Geometry: final body of the model. Coordinates: model frame, mm. A direction names the side the tool comes from. Give positions to 0.01 mm unless a question says otherwise; leave off trailing zeros. Write each loop counter-clockwise with the first axis right and the second up, starting at its lowest first coordinate (ties: lowest second). Pieces come first, ordered by that corner, then holes. Notation, with made-up numbers: M 7.5,-24 L 14.5,-24 A16 cw 14.5,0 Z; hole C -37,59.25 d3. An arc over 180 degrees is marked long. Answer as a JSON object with one key per item and string values.
from build123d import *

# Parameters (mm, degrees)
F0_R      = 14
F1_DEPTH  = 27.75
F5_R      = 4.45
F6_DEPTH  = 2
F7_R      = 1.55
F8_DEPTH  = 5.6
F9_R      = 4.5
F12_DEPTH = 4.7
F13_R     = 1.5
F14_DEPTH = 4.2
F15_R     = 1
F16_DEPTH = 5.5


with BuildPart() as f1:
    # F0 (on Top) → F1 (new body)
    with BuildSketch(Plane.XY):
        Circle(F0_R)
    extrude(amount=F1_DEPTH)

    # F3 (on Front) → F4 (revolve, cut)
    with BuildSketch(Plane.XZ):
        Polygon((14, 27.75), (9.375, 27.75), (14, 22), align=None)
    revolve(axis=Axis((0, 0, 13.875), (0, 0, -1)), mode=Mode.SUBTRACT)

    # F5 (on face) → F6 (join)
    with BuildSketch(Plane.XY.offset(27.75)):
        Circle(F5_R)
    extrude(amount=F6_DEPTH)

    # F7 (on face) → F8 (join)
    with BuildSketch(Plane.XY.offset(29.75)):
        Circle(F7_R)
    extrude(amount=F8_DEPTH)

    # F10 (on Front) → F11 (revolve, cut)
    with BuildSketch(Plane.XZ):
        Polygon((14, 0), (14, 4.1), (12.375, 0), align=None)
    revolve(axis=Axis((0, 0, 13.875), (0, 0, -1)), mode=Mode.SUBTRACT)

    # F9 (on face) → F12 (cut)
    with BuildSketch(Plane(origin=(0, 0, 0), x_dir=(1, 0, 0), z_dir=(0, 0, -1))):
        Circle(F9_R)
    extrude(amount=-F12_DEPTH, mode=Mode.SUBTRACT)

    # F13 (on face) → F14 (cut)
    with BuildSketch(Plane(origin=(0, 0, 0), x_dir=(1, 0, 0), z_dir=(0, 0, -1))):
        with Locations((-5.656854, 5.656854)):
            Circle(F13_R)
        with Locations((6.717514, 6.717514)):
            Circle(F13_R)
        with Locations((5.656854, -5.656854)):
            Circle(F13_R)
        with Locations((-6.717514, -6.717514)):
            Circle(F13_R)
    extrude(amount=-F14_DEPTH, mode=Mode.SUBTRACT)

    # F15 (on face) → F16 (cut)
    with BuildSketch(Plane.XY.offset(27.75)):
        with Locations((0, -6)):
            Circle(F15_R)
        with Locations((6, 0)):
            Circle(F15_R)
        with Locations((0, 6)):
            Circle(F15_R)
        with Locations((-6, 0)):
            Circle(F15_R)
    extrude(amount=-F16_DEPTH, mode=Mode.SUBTRACT)


solid = f1.part
1) Cut plane C-C on z = 25.5. Return loops of the section in (x, y).
Geometry check:
{"outline": "C 0,0 d22.37; hole C -6,0 d2; hole C 0,-6 d2; hole C 0,6 d2; hole C 6,0 d2"}
2) Set-up query: faces 1 (the flat face through (-6, -6, 4.2)), 2 (the flat face through (5, 0, 0)), 3 (the cylindrical face through (0, -5, 25)). Return all of +Z, -Z, +X, -X, +Y, -Y with unobstructed straight access to the full face (end or side cutting, diameter ignored); none if empty.
Geometry check:
{"face 1": "-Z", "face 2": "-Z, +X, -X, +Y, -Y", "face 3": "+Z"}
3) Cut plane A-A on y = 0. Return loops of the section in (x, z) (3 decimals), and give its area (3 significant figures).
Geometry check:
{"outline": "M -14,4.1 L -12.375,0 L -4.5,0 L -4.5,4.7 L 4.5,4.7 L 4.5,0 L 12.375,0 L 14,4.1 L 14,22 L 9.375,27.75 L 7,27.75 L 7,22.25 L 5,22.25 L 5,27.75 L 4.45,27.75 L 4.45,29.75 L 1.55,29.75 L 1.55,35.35 L -1.55,35.35 L -1.55,29.75 L -4.45,29.75 L -4.45,27.75 L -5,27.75 L -5,22.25 L -7,22.25 L -7,27.75 L -9.375,27.75 L -14,22 Z", "area": "715 mm2"}
4) Contact query for flat-ended pins moving along their axis: P1, Ø1.8, axis at x = 0, y = 6, coming from the +Z side; P2, Ø2.5, axis at x = -6, y = 0, coming from the +Z side; P3, Ø2, axis at x = -7.5, z = 7.5, coming from the +Y side; P4, Ø5, axis at x = 10, z = 30.5, coming from the +Y side. Output: stop coordinate, or through.
Geometry check:
{"P1": "stops at z = 22.25", "P2": "stops at z = 27.75", "P3": "stops at y = 12.4", "P4": "passes through"}
5) Cut plane D-D on z = 10.5. Return loops of the section in (x, y).
Geometry check:
{"outline": "C 0,0 d28"}
6) Line query: line 1 (Y direction, x = 0, z = 17.5); line 2 (Y direction, x = -1.5, z = 3); line 3 (Y direction, x = 0, z = 2.55). Output: solid intervals per line, ascending. Write a range as from..to.
Geometry check:
{"line 1": "y = -14..14", "line 2": "y = -13.48..-4.24, 4.24..13.48", "line 3": "y = -13.39..-4.5, 4.5..13.39"}
7) Pull-direction query (X, two-part tool) for faces 4 (the flat face through (6, 0, 22.25)), 5 (the flat face through (0, 0, 35.35)), 6 (the conical face through (-2.095, 9.435, 27.39)); classes: pulls with the +X half, pulls with the -X half, needs draft (parallel to the pull), parting line crosses it, or undercut.
Geometry check:
{"face 4": "undercut", "face 5": "needs draft", "face 6": "parting line crosses it"}
